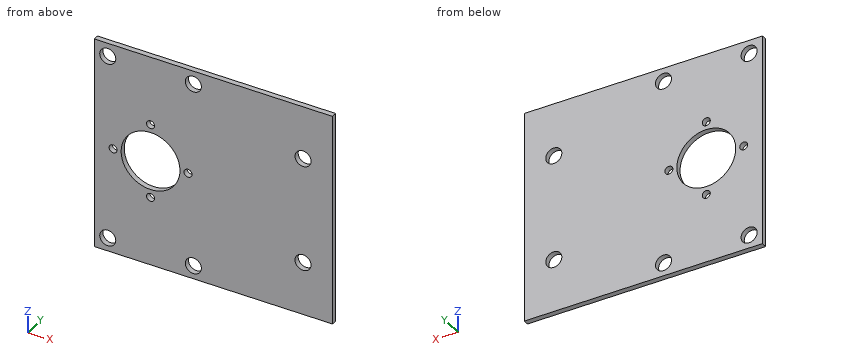
from build123d import *

# Parameters (mm, degrees)
ESQUISSE1_W      = 89
ESQUISSE1_H      = 80
EXTRUSION1_DEPTH = 2
ESQUISSE2_R      = 11
EXTRUSION3_DEPTH = 120.687092036
ESQUISSE4_R      = 1.5
ESQUISSE4_R_2    = 3
EXTRUSION4_DEPTH = 120.687092036


with BuildPart() as part:
    # Esquisse1 → Extrusion1 (new body)
    with BuildSketch(Plane(origin=(0, 0, 0), x_dir=(1, 0, 0), z_dir=(0, 1, 0))):
        with Locations((44.5, 40)):
            Rectangle(ESQUISSE1_W, ESQUISSE1_H)
    extrude(amount=EXTRUSION1_DEPTH)

    # Esquisse2 → Extrusion3 (cut, through all)
    with BuildSketch(Plane(origin=(0, 2, 0), x_dir=(1, 0, 0), z_dir=(0, 1, 0))):
        with Locations(Location((21, 40, 0), (0, 0, 270))):
            Circle(ESQUISSE2_R)
    extrude(amount=-EXTRUSION3_DEPTH, mode=Mode.SUBTRACT)

    # Esquisse4 → Extrusion4 (cut, through all)
    with BuildSketch(Plane(origin=(0, 2, 0), x_dir=(-1, 0, 0), z_dir=(0, 1, 0))):
        with Locations(Location((-35, -40, 0), (0, 0, 90))):
            Circle(ESQUISSE4_R)
        with Locations(Location((-21, -26, 0), (0, 0, 90))):
            Circle(ESQUISSE4_R)
        with Locations(Location((-7, -40, 0), (0, 0, 90))):
            Circle(ESQUISSE4_R)
        with Locations(Location((-21, -54, 0), (0, 0, 90))):
            Circle(ESQUISSE4_R)
        with Locations(Location((-5, -75, 0), (0, 0, 90))):
            Circle(ESQUISSE4_R_2)
        with Locations(Location((-5, -5, 0), (0, 0, 270))):
            Circle(ESQUISSE4_R_2)
        with Locations(Location((-37, -5, 0), (0, 0, 90))):
            Circle(ESQUISSE4_R_2)
        with Locations(Location((-37, -75, 0), (0, 0, 270))):
            Circle(ESQUISSE4_R_2)
        with Locations(Location((-78, -60, 0), (0, 0, 90))):
            Circle(ESQUISSE4_R_2)
        with Locations(Location((-78, -20, 0), (0, 0, 270))):
            Circle(ESQUISSE4_R_2)
    extrude(amount=-EXTRUSION4_DEPTH, mode=Mode.SUBTRACT)


solid = part.part
Could you check a few things on this model? Use its own coordinates, in mm. Round coordinates to 2 decimals unless told otherwise and drop trailing zeros. Write each loop counter-clockwise with the first axis right and the second up, starting at its lowest first coordinate (ties: lowest second). Pieces come first, ordered by that corner, then holes. Notation, with made-up numbers: (-17, -31) -> (38, -31) arc R22 ccw to (38, 5) -> close; hole circle Ø8 at (-15.5, 19.5). An arc over 180 degrees is marked (long way). Use a Markdown table: item, result.
1. For pin 1 Ø3.5 at (x, z) = (5, -75) entering from +Y, with a flat end and sliding along its axis, tell me the tip position at first contact or that it passes through.
Answer key:
| item | result |
|---|---|
| pin 1 | passes through |
2. If we section it at A-A (x = 78): List the corners of the cut face in (y, z) for me, then the cut area to 3 significant figures.
Answer key:
| item | result |
|---|---|
| outline | (0, -80) -> (2, -80) -> (2, -63) -> (0, -63) -> close; (0, -57) -> (2, -57) -> (2, -23) -> (0, -23) -> close; (0, -17) -> (2, -17) -> (2, 0) -> (0, 0) -> close |
| area | 136 mm^2 |
3. If we section it at B-B (z = -40): List the corners of the cut face in (x, y) for me.
Answer key:
| item | result |
|---|---|
| outline | (0, 0) -> (5.5, 0) -> (5.5, 2) -> (0, 2) -> close; (8.5, 0) -> (10, 0) -> (10, 2) -> (8.5, 2) -> close; (32, 0) -> (33.5, 0) -> (33.5, 2) -> (32, 2) -> close; (36.5, 0) -> (89, 0) -> (89, 2) -> (36.5, 2) -> close |
4. If we section it at C-C (y = 0.45): State how many separate pieces and enclosed holes the cut face has, then the cut area to 3 significant figures.
Answer key:
| item | result |
|---|---|
| separate pieces | 1 |
| enclosed holes | 11 |
| area | 6,540 mm^2 |
5. If we section it at D-D (x = 21): List the corners of the cut face in (y, z) for me, then the cut area to 3 significant figures.
Answer key:
| item | result |
|---|---|
| outline | (0, -80) -> (2, -80) -> (2, -55.5) -> (0, -55.5) -> close; (0, -52.5) -> (2, -52.5) -> (2, -51) -> (0, -51) -> close; (0, -29) -> (2, -29) -> (2, -27.5) -> (0, -27.5) -> close; (0, -24.5) -> (2, -24.5) -> (2, 0) -> (0, 0) -> close |
| area | 104 mm^2 |
6. Please list where these lines run through material, in increasing order: probe 1 along X at (y, z) = (0.35, -75); probe 2 along X at (y, z) = (0.4, -40); probe 3 along Z at (x, y) = (79.5, 0.8).
Answer key:
| item | result |
|---|---|
| probe 1 | x = 0 to 2, 8 to 34, 40 to 89 |
| probe 2 | x = 0 to 5.5, 8.5 to 10, 32 to 33.5, 36.5 to 89 |
| probe 3 | z = -80 to -62.6, -57.4 to -22.6, -17.4 to 0 |
